Input: dimensioned drawing with shaded views. Units: mm. Origin: part minimum x, y, z. Round coordinates to 2 decimals unless told otherwise and drop trailing zeros. Write each loop counter-clockwise with the first axis right and the second up, starting at its lowest first coordinate (ties: lowest second). Pieces come first, ordered by that corner, then holes. Notation, with made-up numbers: M 30.25,-38 L 86.25,-38 A21 cw 86.25,-13 Z; hole C 85.25,45 d5. An arc over 180 degrees is marked long. Use one line per item in the form item = value. Start each with the question number.
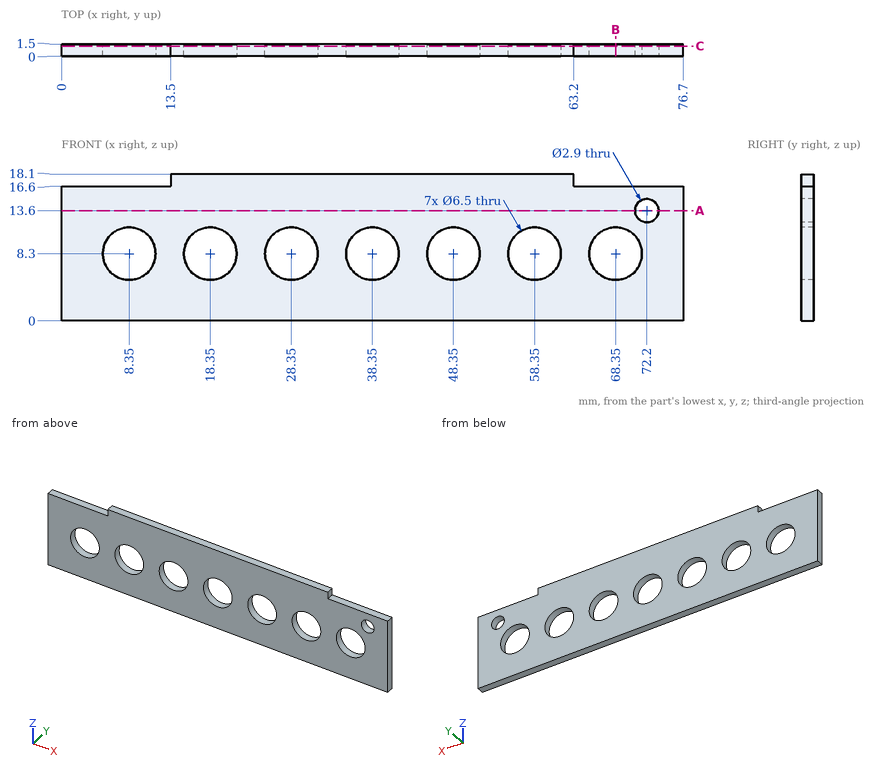
1. Contact query for a flat-ended pin moving along its axis: pin 1 (0.8 mm diameter, centred on x = 71, y = 1, fed in from +Z). Output: stop coordinate, or through.
2. Ray query, probe 1 along Z at (x, y) = (18.35, 1.05); probe 2 along Z at (x, y) = (68.35, 0.55); probe 3 along X at (y, z) = (0.95, 17.5). Return the intervals inside material, ascending.
3. Section query B-B (x = 68.35). Return loops of the section in (y, z), then the cut area to 4 significant figures.
4. Section query A-A (z = 13.6). Return loops of the section in (x, y), then the cut area to 3 significant figures.
5. Section query C-C (y = 1.25). Give the number of separate pieces and of enclosed holes in the cut face, then the cut area to 3 significant figures.
Checks:
q1.pin_1 = 16.6
q2.probe_1 = 0 to 5.05, 11.55 to 18.1
q2.probe_2 = 0 to 5.05, 11.55 to 16.6
q2.probe_3 = 13.5 to 63.2
q3.outline = M 0,0 L 1.5,0 L 1.5,5.05 L 0,5.05 Z; M 0,11.55 L 1.5,11.55 L 1.5,16.6 L 0,16.6 Z
q3.area = 15.15 mm^2
q4.outline = M 0,0 L 70.75,0 L 70.75,1.5 L 0,1.5 Z; M 73.65,0 L 76.7,0 L 76.7,1.5 L 73.65,1.5 Z
q4.area = 111 mm^2
q5.separate_pieces = 1
q5.enclosed_holes = 8
q5.area = 1,110 mm^2
